```python
from build123d import *

# Parameters (mm, degrees)
SKETCH1_W           = 203.2
SKETCH1_H           = 50.8
BOSS_EXTRUDE1_DEPTH = 12.7
CUT_EXTRUDE1_DEPTH  = 115.3
SKETCH4_R           = 2.38125
CUT_EXTRUDE3_DEPTH  = 106.494123059
LPATTERN1_COUNT     = 5
LPATTERN1_PITCH     = 38.1
SKETCH5_R           = 3.175
CUT_EXTRUDE4_DEPTH  = 12.7


with BuildPart() as part:
    # Sketch1 → Boss-Extrude1 (new body)
    with BuildSketch(Plane(origin=(0, 0, 0), x_dir=(0, 0, -1), z_dir=(1, 0, 0))):
        Rectangle(SKETCH1_W, SKETCH1_H)
    extrude(amount=BOSS_EXTRUDE1_DEPTH)

    # Sketch2 → Cut-Extrude1 (cut, through all)
    with BuildSketch(Plane(origin=(0, 25.4, 0), x_dir=(1, 0, 0), z_dir=(0, 1, 0))):
        Polygon((0, 101.6), (12.7, 88.9), (12.7, 101.6), align=None)
        Polygon((0, -101.6), (12.7, -88.9), (12.7, -101.6), align=None)
    extrude(amount=-CUT_EXTRUDE1_DEPTH, mode=Mode.SUBTRACT)

    # Sketch4 → Cut-Extrude3 (cut, through all)
    with BuildSketch(Plane.ZY):
        with Locations((-76.2, -19.05)):
            Circle(SKETCH4_R)
    cut_extrude3 = extrude(amount=-CUT_EXTRUDE3_DEPTH, mode=Mode.SUBTRACT)

    # LPattern1: Cut-Extrude3 ×5
    with Locations(*[(0, 0, i * LPATTERN1_PITCH) for i in range(1, LPATTERN1_COUNT)]):
        add(cut_extrude3, mode=Mode.SUBTRACT)

    # Sketch5 → Cut-Extrude4 (cut)
    with BuildSketch(Plane(origin=(0, 25.4, 0), x_dir=(1, 0, 0), z_dir=(0, 1, 0))):
        with Locations(Location((6.35, 76.2, 0), (0, 0, 270))):
            Circle(SKETCH5_R)
        with Locations(Location((6.35, -76.2, 0), (0, 0, 270))):
            Circle(SKETCH5_R)
    extrude(amount=-CUT_EXTRUDE4_DEPTH, mode=Mode.SUBTRACT)


solid = part.part
```
Check sheet for the modelled part. Datum: model origin and axes. Units: mm. A direction names the side the tool comes from. Coordinates: 2 decimals unless noted, no trailing zeros. Order: outer loops, then holes, each group sorted by start corner. A loop starts at its lowest first (then second) coordinate and runs counter-clockwise, first axis right, second up. Notation, with made-up numbers: M 58,-15.5 L 96,-15.5 A12 ccw 96,0.5 Z; hole C 48,42 d8. An arc over 180 degrees is marked long. Write each question's results on one line, items separated by ' | '. Start each with the question number.
1. Go/stop test with flat-tipped pins: P1, Ø1.5, axis at x = 8.5, y = 4, coming from the -Z side; P2, Ø3, axis at y = 13, z = -76, coming from the -X side. Record where each tip stops, or that it passes through.
2. Cross-section at D-D on z = 38.1. Record the cut outline in (x, y), and give its area (3 significant figures).
3. Cross-section at B-B on y = -19.05. Record the cut outline in (x, z), and give its area (3 significant figures).
4. Cross-section at A-A on z = -76.2. Record the cut outline in (x, y) (3 decimals).
5. Material ranges on probe 1 along Y at (x, z) = (2, 76.5); probe 2 along Y at (x, z) = (4.75, -76.2); probe 3 along Z at (x, y) = (5.5, 17.5), recorded low to high.
6. Access from +Z, -Z, +X, -X, +Y, -Y to the whole of each face (thin tool, end or side, straight path). Record for faces 1 (the face through (0, 0, 1)), 2 (the face through (7.3, 19.14, -73.17)).
7. Mould release check, pull along Y, two halves, no side actions. Record for faces 3 (the face through (6.3, 0.4, -95.3)), 4 (the face through (6.26, -18.95, -40.48)), 5 (the face through (6.26, -21.16, -75.1)), 6 (the face through (6, 25.4, 1)): +Y half, -Y half, draft (parallel to the pull), parting line (faces both ways), or undercut.
8. Cross-section at C-C on x = 6.35. State how many separate pieces and enclosed holes the cut face has, and give its area (3 significant figures).
Checks:
1) P1: stops at z = -93.85 | P2: stops at x = 0
2) outline: M 0,-25.4 L 12.7,-25.4 L 12.7,-21.43 L 0,-21.43 Z; M 0,-16.67 L 12.7,-16.67 L 12.7,25.4 L 0,25.4 Z | area: 585 mm²
3) outline: M 0,-101.6 L 12.7,-88.9 L 12.7,-78.58 L 0,-78.58 Z; M 0,-73.82 L 12.7,-73.82 L 12.7,-40.48 L 0,-40.48 Z; M 0,-35.72 L 12.7,-35.72 L 12.7,-2.38 L 0,-2.38 Z; M 0,2.38 L 12.7,2.38 L 12.7,35.72 L 0,35.72 Z; M 0,40.48 L 12.7,40.48 L 12.7,73.82 L 0,73.82 Z; M 0,78.58 L 12.7,78.58 L 12.7,88.9 L 0,101.6 Z | area: 2,120 mm²
4) outline: M 0,-25.4 L 12.7,-25.4 L 12.7,-21.431 L 0,-21.431 Z; M 0,-16.669 L 12.7,-16.669 L 12.7,25.4 L 9.525,25.4 L 9.525,12.7 L 3.175,12.7 L 3.175,25.4 L 0,25.4 Z
5) probe 1: y = -25.4 to -21.41, -16.69 to 25.4 | probe 2: y = -25.4 to -21.43, -16.67 to 12.7 | probe 3: z = -96.1 to -79.26, -73.14 to 73.14, 79.26 to 96.1
6) face 1: +Z, -Z, -X, +Y, -Y | face 2: +Y
7) face 3: draft | face 4: undercut | face 5: undercut | face 6: +Y half
8) separate pieces: 1 | enclosed holes: 5 | area: 9,430 mm²
